Study the drawing (mm; zero at the part's minimum x, y, z) and answer. A direction names the side the tool comes from. Round coordinates to 2 decimals unless told otherwise and drop trailing zeros. Order: outer loops, then holes, each group sorted by start corner. A loop starts at its lowest first (then second) coordinate and runs counter-clockwise, first axis right, second up. Notation, with made-up numbers: (87, 12) - (140, 12) arc R18 ccw to (140, 47) - close; hole circle Ø4 at (-11.5, 80.25). An arc over 180 degrees is marked (long way). Put each result on its own line as item: value. Start each with the question number.
Q1. Section A-A on x = 7.5 is taken. Give the vertices of the cut face in (y, z).
Q2. Section D-D on y = 27.5 is taken. Give the vertices of the cut face in (x, z), then the cut area to 3 significant figures.
Q3. Each of these flat-tipped pins is pushed along its axis until it touches: pin 1 Ø2 at (y, z) = (20.5, 3) entering from +X; pin 2 Ø2 at (x, y) = (9.5, 24) entering from -Z; pin 3 Ø3 at (x, y) = (8.5, 28.5) entering from -Z. Where does it stop, or does it pass through?
Q4. For a pull along Y with two mould halves and no side action, classify the marked faces 3, 4 and 5 as pulls with the +Y half, pulls with the -Y half, needs draft (parallel to the pull), parting line crosses it, or undercut.
Q5. Which of the six approach directions +Z, -Z, +X, -X, +Y, -Y give full straight-line access (tool end or side, diameter ignored) to the marked faces 1 and 2?
Q6. Section B-B on z = 1.5 is taken. Give the vertices of the cut face in (x, y).
Q7. Find the intervals of material crossed by line 1 along Y through (x, z) = (7.5, 0.85); line 2 along Y through (x, z) = (3, 4.75); line 3 along X through (y, z) = (27.5, 1.6), in increasing order. Write a range as from..to.
Q8. Section C-C on y = 17.5 is taken. Give the vertices of the cut face in (x, z).
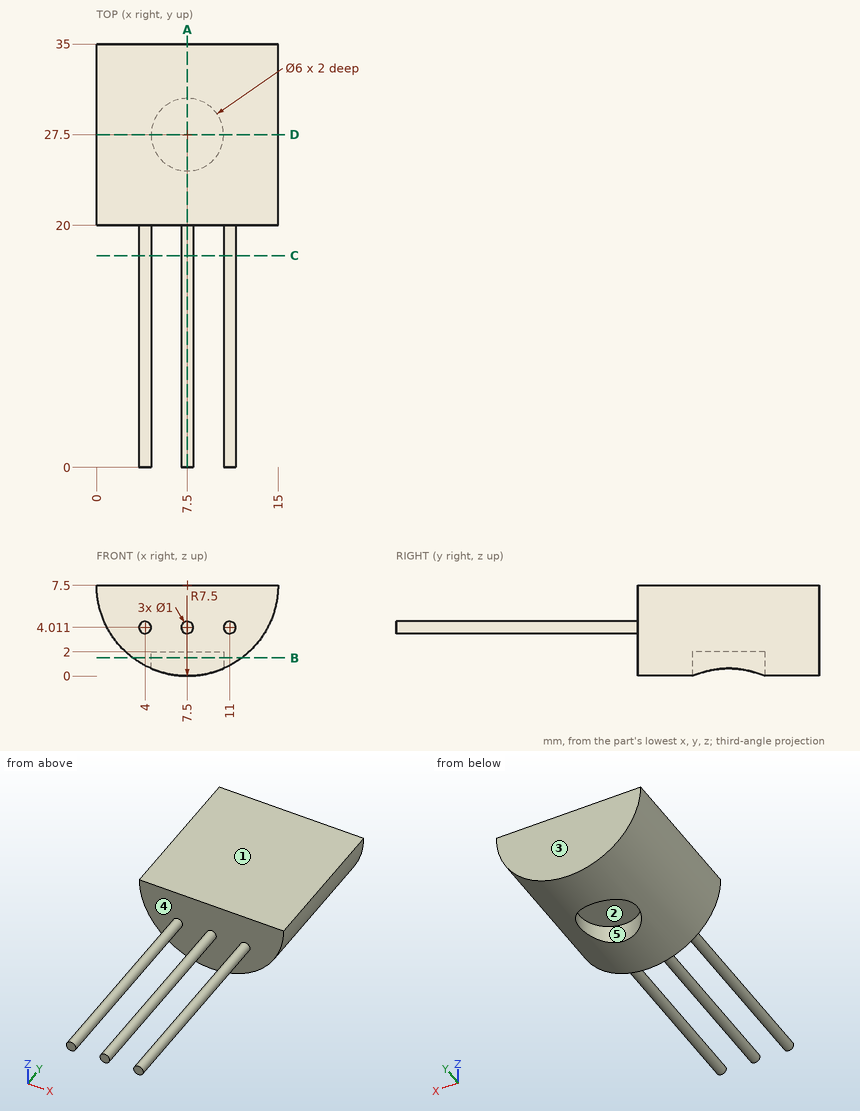
Findings:
1. outline: (0, 3.51) - (20, 3.51) - (20, 0) - (24.5, 0) - (24.5, 2) - (30.5, 2) - (30.5, 0) - (35, 0) - (35, 7.5) - (20, 7.5) - (20, 4.51) - (0, 4.51) - close
2. outline: (0, 7.5) arc R7.5 ccw to (4.5, 0.63) - (4.5, 2) - (10.5, 2) - (10.5, 0.63) arc R7.5 ccw to (15, 7.5) - close
2. area: 77.6 mm2
3. pin 1: x = 14.13
3. pin 2: z = 0.07
3. pin 3: z = 2
4. face 3: pulls with the +Y half
4. face 4: pulls with the -Y half
4. face 5: undercut
5. face 1: +Z, +X, -X, +Y, -Y
5. face 2: -Z
6. outline: (3, 20) - (12, 20) - (12, 35) - (3, 35) - close; hole circle Ø6 at (7.5, 27.5)
7. line 1: 20..24.5, 30.5..35
7. line 2: 20..35
7. line 3: 2.87..4.5, 10.5..12.13
8. outline: circle Ø1 at (4, 4.01); circle Ø1 at (7.5, 4.01); circle Ø1 at (11, 4.01)
